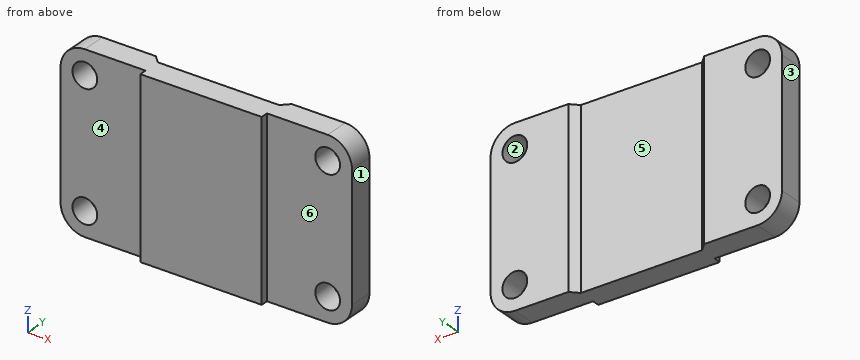
from build123d import *

# Parameters (mm, degrees)
SKETCH1_W              = 120
SKETCH1_H              = 72
BOSS_EXTRUDE1_DEPTH    = 10
FILLET1_R              = 10
M12_TAPPED_HOLE1_D     = 10.2
M12_TAPPED_HOLE1_DEPTH = 10
SKETCH6_W              = 50
SKETCH6_H              = 72
BOSS_EXTRUDE2_DEPTH    = 3
CUT_EXTRUDE1_DEPTH     = 73


with BuildPart() as part:
    # Sketch1 → Boss-Extrude1 (new body)
    with BuildSketch(Plane(origin=(0, 0, 0), x_dir=(1, 0, 0), z_dir=(0, 1, 0))):
        Rectangle(SKETCH1_W, SKETCH1_H)
    extrude(amount=BOSS_EXTRUDE1_DEPTH)

    # Fillet1
    fillet1_edges = [part.edges().sort_by_distance(p)[0] for p in [
        (60, 5, 36),
        (-60, 5, 36),
        (-60, 5, -36),
        (60, 5, -36),
    ]]
    fillet(fillet1_edges, radius=FILLET1_R)

    # M12 Tapped Hole1
    with Locations(Plane.XZ):
        with Locations((50, -26), (50, 26), (-50, 26), (-50, -26)):
            Hole(M12_TAPPED_HOLE1_D / 2, depth=M12_TAPPED_HOLE1_DEPTH)

    # Sketch6 → Boss-Extrude2 (add)
    with BuildSketch(Plane(origin=(0, 0, 0), x_dir=(1, 0, 0), z_dir=(0, 1, 0))):
        Rectangle(SKETCH6_W, SKETCH6_H)
    extrude(amount=-BOSS_EXTRUDE2_DEPTH)

    # Sketch11 → Cut-Extrude1 (cut, through all)
    with BuildSketch(Plane.XY.offset(36)):
        Polygon((-28, 10), (-25, 7), (25, 7), (28, 10), align=None)
    extrude(amount=-CUT_EXTRUDE1_DEPTH, mode=Mode.SUBTRACT)


solid = part.part
Work out the finished part from the listing and answer in its coordinate system (mm). Face numbers are marked on the shaded views. A direction names the side the tool comes from. Give positions to 0.01 mm unless a question says otherwise; leave off trailing zeros. Write each loop counter-clockwise with the first axis right and the second up, starting at its lowest first coordinate (ties: lowest second). Pieces come first, ordered by that corner, then holes.
Q1. Straight lines are drawn through the part: L1, parallel to Z at x = -50, y = 7; L2, parallel to Z at x = 54, y = 6.75; L3, parallel to Y at x = -39, z = -27. For each, find the intervals that lie inside material, in ascending order.
Answer:
L1: z = -36 to -31.1, -20.9 to 20.9, 31.1 to 36
L2: z = -35.17 to -29.16, -22.84 to 22.84, 29.16 to 35.17
L3: y = 0 to 10
Q2. Given pin 1 (10 mm diameter, centred on x = -21, z = -1, fed in from +Y); pin 2 (0.9 mm diameter, centred on y = -1.5, z = 10, fed in from -X); pin 3 (1.5 mm diameter, centred on y = -1, z = 9, fed in from +X); pin 4 (16.5 mm diameter, centred on x = -50, z = -26, fed in from +Y), each flat-ended and moving along its own axis, determine where each tip first touches the part or whether it passes through.
Answer:
pin 1: stops at y = 8
pin 2: stops at x = -25
pin 3: stops at x = 25
pin 4: stops at y = 10
Q3. For a pull along X with two mould halves and no side action, classify the marked faces 1, 2 and 3 as released by +X, released by -X, zero draft, split by the parting line, or undercut.
Answer:
face 1: released by +X
face 2: undercut
face 3: released by -X
Q4. The part is cut by section C-C on z = -24.5. Give the vertices of the cut face in (x, y), and give its area (3 significant figures).
Answer:
outline: (-60, 0) - (-54.87, 0) - (-54.87, 10) - (-60, 10) - close; (-45.13, 0) - (-25, 0) - (-25, -3) - (25, -3) - (25, 0) - (45.13, 0) - (45.13, 10) - (28, 10) - (25, 7) - (-25, 7) - (-28, 10) - (-45.13, 10) - close; (54.87, 0) - (60, 0) - (60, 10) - (54.87, 10) - close
area: 996 mm2
Q5. The part is cut by section A-A on x = 51.5. Give the vertices of the cut face in (y, z), and give its area (3 significant figures).
Answer:
outline: (0, -35.89) - (10, -35.89) - (10, -30.87) - (0, -30.87) - close; (0, -21.13) - (10, -21.13) - (10, 21.13) - (0, 21.13) - close; (0, 30.87) - (10, 30.87) - (10, 35.89) - (0, 35.89) - close
area: 523 mm2
Q6. The part is cut by section B-B on y = 2.75. Give the vertices of the cut face in (x, z), and give its area (3 significant figures).
Answer:
outline: (-60, -26) arc R10 ccw to (-50, -36) - (50, -36) arc R10 ccw to (60, -26) - (60, 26) arc R10 ccw to (50, 36) - (-50, 36) arc R10 ccw to (-60, 26) - close; hole circle Ø10.2 at (-50, -26); hole circle Ø10.2 at (-50, 26); hole circle Ø10.2 at (50, -26); hole circle Ø10.2 at (50, 26)
area: 8,230 mm2
Q7. The part is cut by section D-D on x = 19. Give the vertices of the cut face in (y, z), and give its area (3 significant figures).
Answer:
outline: (-3, -36) - (7, -36) - (7, 36) - (-3, 36) - close
area: 720 mm2
Q8. A tool of negligible diameter and unlimited length cuts with its end or side. For the marked faces 4, 5 and 6, from which of +Z, -Z, +X, -X, +Y, -Y can it reach the whole face along a straight path? Write none if from no direction.
Answer:
face 4: +Z, -Z, -X, -Y
face 5: +Z, -Z, +Y
face 6: +Z, -Z, +X, -Y
